The drawing under review shows one solid part. Ordinate dimensions are in mm from its lowest x, y, z. A direction names the side the tool comes from. Round coordinates to 2 decimals unless told otherwise and drop trailing zeros. Order: outer loops, then holes, each group sorted by start corner. A loop starts at its lowest first (then second) coordinate and runs counter-clockwise, first axis right, second up.
1) Mouldability with a two-part tool opening along Z and no side actions: class the marked faces 3, 4 and 5 as pulls with the +Z half, pulls with the -Z half, needs draft (parallel to the pull), parting line crosses it, or undercut.
2) Consider section A-A (y = 2.5). Give the boundary of the cut face in (x, z).
3) Consider section D-D (z = 22.5). Give the boundary of the cut face in (x, y).
4) Consider section C-C (x = 15). Give the boundary of the cut face in (y, z), then the cut area to 3 significant figures.
5) Consider section B-B (z = 17). Give the boundary of the cut face in (x, y), then the cut area to 3 significant figures.
6) Clearance check with flat-ended pins moving along their axes: P1, Ø8.5, axis at x = 21, z = 12.5, coming from the +Y side; P2, Ø4, axis at x = 31, z = 3, coming from the -Y side; P3, Ø3.5, axis at x = 17, z = 17, coming from the +Y side. State where each tip first meets the part, or that it passes through.
7) To check wall thickness, follow L1, parallel to X at y = 0.95, z = 17; L2, parallel to X at y = 6.75, z = 9.5; L3, parallel to X at y = 4.5, z = 32. State the ranges of each line that lie inside material, in increasing order.
8) Machinability: for the marked faces 1 and 2, which of the approach directions +Z, -Z, +X, -X, +Y, -Y give a long, thin tool a straight path to every point of the face, cutting with its end or side? Answer none if there is none.
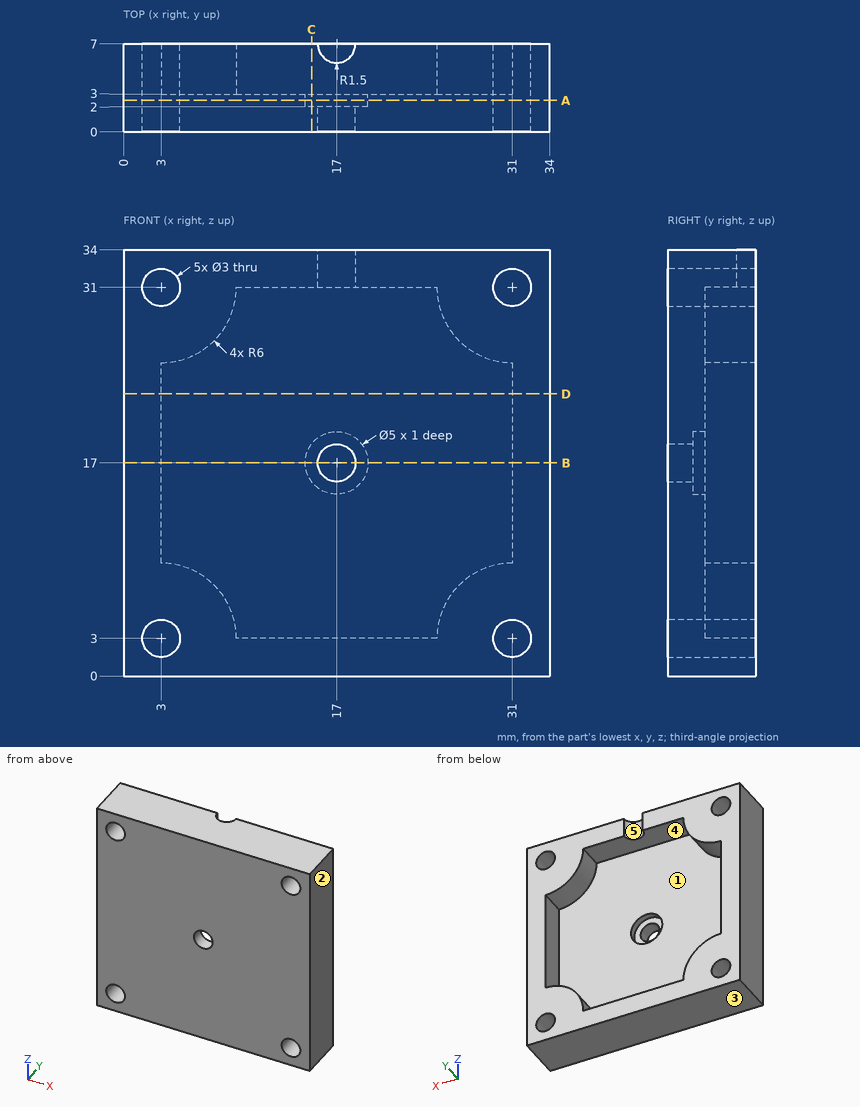
Answer below:
1. face 3: pulls with the -Z half
1. face 4: undercut
1. face 5: needs draft
2. outline: (0, 0) - (34, 0) - (34, 34) - (0, 34) - close; hole circle Ø3 at (3, 3); hole circle Ø3 at (3, 31); hole circle Ø5 at (17, 17); hole circle Ø3 at (31, 3); hole circle Ø3 at (31, 31)
3. outline: (0, 0) - (34, 0) - (34, 7) - (31, 7) - (31, 3) - (3, 3) - (3, 7) - (0, 7) - close
4. outline: (0, 0) - (7, 0) - (7, 3) - (3, 3) - (3, 15.5) - (2, 15.5) - (2, 18.5) - (3, 18.5) - (3, 31) - (7, 31) - (7, 34) - (0, 34) - close
4. area: 123 mm2
5. outline: (0, 0) - (15.5, 0) - (15.5, 2) - (14.5, 2) - (14.5, 3) - (3, 3) - (3, 7) - (0, 7) - close; (18.5, 0) - (34, 0) - (34, 7) - (31, 7) - (31, 3) - (19.5, 3) - (19.5, 2) - (18.5, 2) - close
5. area: 115 mm2
6. P1: stops at y = 3
6. P2: stops at y = 0
6. P3: stops at y = 2
7. L1: x = 0 to 15.5, 18.5 to 34
7. L2: x = 0 to 3, 31 to 34
7. L3: x = 0 to 1.88, 4.12 to 29.88, 32.12 to 34
8. face 1: +Y
8. face 2: +Z, -Z, +X, +Y, -Y
